```python
from build123d import *

# Parameters (mm, degrees)
SKETCH1_W                                            = 40
SKETCH1_H                                            = 36
BOSS_EXTRUDE1_DEPTH                                  = 5
SKETCH2_R                                            = 4
CUT_EXTRUDE1_DEPTH                                   = 28.367864367
CSK_FOR_M2_5_COUNTERSUNK_FLAT_HEAD_SCREW_D           = 2.9
CSK_FOR_M2_5_COUNTERSUNK_FLAT_HEAD_SCREW_CSINK_D     = 5.5
CSK_FOR_M2_5_COUNTERSUNK_FLAT_HEAD_SCREW_CSINK_ANGLE = 90
CSK_FOR_M2_COUNTERSUNK_FLAT_HEAD_SCREW1_D            = 2.4
CSK_FOR_M2_COUNTERSUNK_FLAT_HEAD_SCREW1_CSINK_D      = 4.4
CSK_FOR_M2_COUNTERSUNK_FLAT_HEAD_SCREW1_CSINK_ANGLE  = 90


with BuildPart() as part:
    # Sketch1 → Boss-Extrude1 (new body)
    with BuildSketch(Plane(origin=(0, 0, 0), x_dir=(1, 0, 0), z_dir=(0, 1, 0))):
        Rectangle(SKETCH1_W, SKETCH1_H)
    extrude(amount=BOSS_EXTRUDE1_DEPTH)

    # Sketch2 → Cut-Extrude1 (cut, through all)
    with BuildSketch(Plane(origin=(0, 5, 0), x_dir=(1, 0, 0), z_dir=(0, 1, 0))):
        with Locations(Location((0, 0, 0), (0, 0, 270))):
            Circle(SKETCH2_R)
    extrude(amount=-CUT_EXTRUDE1_DEPTH, mode=Mode.SUBTRACT)

    # CSK for M2.5 Countersunk Flat Head Screw1 (through all)
    with Locations(Plane(origin=(0, 5, 0), x_dir=(1, 0, 0), z_dir=(0, 1, 0))):
        with Locations((-7.5, 0), (7.5, 0)):
            CounterSinkHole(CSK_FOR_M2_5_COUNTERSUNK_FLAT_HEAD_SCREW_D / 2, CSK_FOR_M2_5_COUNTERSUNK_FLAT_HEAD_SCREW_CSINK_D / 2, counter_sink_angle=CSK_FOR_M2_5_COUNTERSUNK_FLAT_HEAD_SCREW_CSINK_ANGLE)

    # CSK for M2 Countersunk Flat Head Screw1 (through all)
    with Locations(Plane(origin=(0, 0, 0), x_dir=(-1, 0, 0), z_dir=(0, -1, 0))):
        with Locations((17.5, -7.5), (17.5, 7.5), (-17.5, 7.5), (-17.5, -7.5)):
            CounterSinkHole(CSK_FOR_M2_COUNTERSUNK_FLAT_HEAD_SCREW1_D / 2, CSK_FOR_M2_COUNTERSUNK_FLAT_HEAD_SCREW1_CSINK_D / 2, counter_sink_angle=CSK_FOR_M2_COUNTERSUNK_FLAT_HEAD_SCREW1_CSINK_ANGLE)


solid = part.part
```
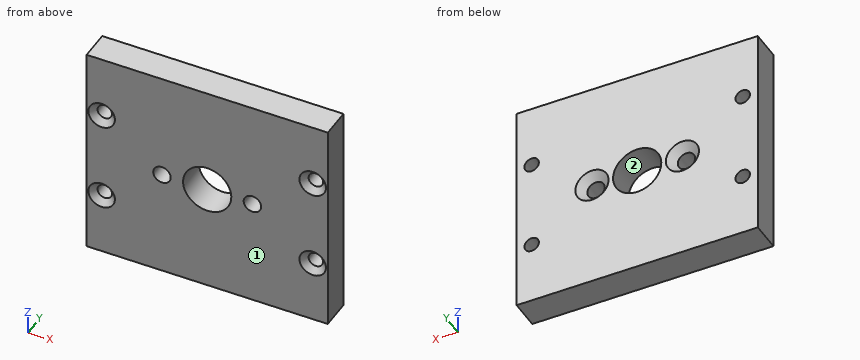
Work out the finished part from the listing and answer in its coordinate system (mm). Face numbers are marked on the shaded views. Give positions to 0.01 mm unless a question says otherwise; leave off trailing zeros. Write each loop counter-clockwise with the first axis right and the second up, starting at its lowest first coordinate (ties: lowest second). Pieces come first, ordered by that corner, then holes.
(1) The mould has two halves that part along X. Classify the marked faces 1 and 2: pulls with the +X half, pulls with the -X half, needs draft (parallel to the pull), parting line crosses it, or undercut.
Final values:
face 1: needs draft
face 2: undercut
(2) The part is cut by section B-B on z = 7.5. Write down the section's boundary in (x, y).
Final values:
outline: (-20, 0) - (-19.7, 0) - (-18.7, 1) - (-18.7, 5) - (-20, 5) - close; (-16.3, 1) - (-15.3, 0) - (15.3, 0) - (16.3, 1) - (16.3, 5) - (-16.3, 5) - close; (18.7, 1) - (19.7, 0) - (20, 0) - (20, 5) - (18.7, 5) - close
(3) The part is cut by section A-A on x = -7.5. Write down the section's boundary in (y, z).
Final values:
outline: (0, -18) - (5, -18) - (5, -2.75) - (3.7, -1.45) - (0, -1.45) - close; (0, 1.45) - (3.7, 1.45) - (5, 2.75) - (5, 18) - (0, 18) - close
(4) Flat-ended cylindrical pins translate along their axes: pin 1 Ø4 at (x, z) = (-7.5, 0) entering from -Y; pin 2 Ø4 at (x, z) = (7.5, 0) entering from +Y; pin 3 Ø4 at (x, z) = (17.5, -7.5) entering from -Y. Find the tip coordinate at first contact, or state that the pin passes through.
Final values:
pin 1: stops at y = 0
pin 2: stops at y = 4.25
pin 3: stops at y = 0.2
(5) Straight lines are drawn through the part: line 1 (X direction, y = 3.25, z = -7.5); line 2 (Z direction, x = 17.5, y = 2.4); line 3 (X direction, y = 0.9, z = 7.5). For each, find the intervals that lie inside material, in ascending order.
Final values:
line 1: x = -20 to -18.7, -16.3 to 16.3, 18.7 to 20
line 2: z = -18 to -8.7, -6.3 to 6.3, 8.7 to 18
line 3: x = -20 to -18.8, -16.2 to 16.2, 18.8 to 20
(6) The part is cut by section D-D on x = 17.5. Write down the section's boundary in (y, z), plus the area to 3 significant figures.
Final values:
outline: (0, -18) - (5, -18) - (5, -8.7) - (1, -8.7) - (0, -9.7) - close; (0, -5.3) - (1, -6.3) - (5, -6.3) - (5, 6.3) - (1, 6.3) - (0, 5.3) - close; (0, 9.7) - (1, 8.7) - (5, 8.7) - (5, 18) - (0, 18) - close
area: 154 mm2
(7) The part is cut by section C-C on z = 0. Write down the section's boundary in (x, y).
Final values:
outline: (-20, 0) - (-8.95, 0) - (-8.95, 3.7) - (-10.25, 5) - (-20, 5) - close; (-6.05, 0) - (-4, 0) - (-4, 5) - (-4.75, 5) - (-6.05, 3.7) - close; (4, 0) - (6.05, 0) - (6.05, 3.7) - (4.75, 5) - (4, 5) - close; (8.95, 0) - (20, 0) - (20, 5) - (10.25, 5) - (8.95, 3.7) - close
